```python
from build123d import *

# Parameters (mm, degrees)
SKETCH_1_R      = 1.5
SKETCH_1_R_2    = 5
EXTRUDE_1_DEPTH = 1


with BuildPart() as part:
    # 草图1 → 凸台-拉伸1 (new body)
    with BuildSketch(Plane.XY):
        with BuildLine():
            Line((-5, 25), (-5, -25))
            ThreePointArc((-5, -25), (0, -30), (5, -25))
            Line((5, -25), (5, 25))
            ThreePointArc((5, 25), (5.598988732, 30.259631636), (7.987721006, 34.983662814))
            ThreePointArc((7.987721006, 34.983662814), (0, 51), (-7.987721006, 34.983662814))
            ThreePointArc((-7.987721006, 34.983662814), (-5.598988732, 30.259631636), (-5, 25))
        make_face()
        with Locations((0, -25)):
            Circle(SKETCH_1_R, mode=Mode.SUBTRACT)
        with Locations((0, 25)):
            Circle(SKETCH_1_R, mode=Mode.SUBTRACT)
        with Locations((7.5, 41)):
            Circle(SKETCH_1_R, mode=Mode.SUBTRACT)
        with Locations((-7.5, 41)):
            Circle(SKETCH_1_R, mode=Mode.SUBTRACT)
        with Locations((0, 33.5)):
            Circle(SKETCH_1_R, mode=Mode.SUBTRACT)
        with Locations((0, 41)):
            Circle(SKETCH_1_R_2, mode=Mode.SUBTRACT)
        with Locations((0, 48.5)):
            Circle(SKETCH_1_R, mode=Mode.SUBTRACT)
    extrude(amount=EXTRUDE_1_DEPTH)


solid = part.part
```
The model under review builds one solid part; all positions refer to its coordinate system, in mm. Give positions to 0.01 mm unless a question says otherwise; leave off trailing zeros. Loops run counter-clockwise (first coordinate to the right, second up) from the corner with the lowest first, then second, coordinate; pieces in that order, holes last. Notation, with made-up numbers: (31.5, 22) -> (72.5, 22) arc R25 cw to (72.5, 39) -> close; hole circle Ø10 at (-27.75, 61). An arc over 180 degrees is marked (long way). Use CSV: the item, a comma, the result in double quotes.
1. Consider section D-D, the plane x = -3.75. Write out the cut boundary in (y, z).
Result:
outline,"(-28.31, 0) -> (37.69, 0) -> (37.69, 1) -> (-28.31, 1) -> close; (44.31, 0) -> (50.27, 0) -> (50.27, 1) -> (44.31, 1) -> close"
2. Consider section C-C, the plane z = 0.15. Write out the cut boundary in (x, y), then the cut area to 3 significant figures.
Result:
outline,"(-7.99, 34.98) arc R15 cw to (-5, 25) -> (-5, -25) arc R5 ccw to (5, -25) -> (5, 25) arc R15 cw to (7.99, 34.98) arc R10 ccw (long way) to start; hole circle Ø3 at (-7.5, 41); hole circle Ø10 at (0, 41); hole circle Ø3 at (0, -25); hole circle Ø3 at (0, 25); hole circle Ø3 at (0, 33.5); hole circle Ø3 at (0, 48.5); hole circle Ø3 at (7.5, 41)"
area,"805 mm²"
3. Consider section A-A, the plane x = 0. Write out the cut boundary in (y, z), then the cut area to 3 significant figures.
Result:
outline,"(-30, 0) -> (-26.5, 0) -> (-26.5, 1) -> (-30, 1) -> close; (-23.5, 0) -> (23.5, 0) -> (23.5, 1) -> (-23.5, 1) -> close; (26.5, 0) -> (32, 0) -> (32, 1) -> (26.5, 1) -> close; (35, 0) -> (36, 0) -> (36, 1) -> (35, 1) -> close; (46, 0) -> (47, 0) -> (47, 1) -> (46, 1) -> close; (50, 0) -> (51, 0) -> (51, 1) -> (50, 1) -> close"
area,"59.0 mm²"
4. To check wall thickness, follow probe 1 along X at (y, z) = (41.5, 0.4); probe 2 along X at (y, z) = (14.5, 0.8); probe 3 along Y at (x, z) = (-0.75, 0.15). State the ranges of each line that lie inside material, in increasing order. Write a range as from..to.
Result:
probe 1,"x = -9.99..-8.91, -6.09..-4.97, 4.97..6.09, 8.91..9.99"
probe 2,"x = -5..5"
probe 3,"y = -29.94..-26.3, -23.7..23.7, 26.3..32.2, 34.8..36.06, 45.94..47.2, 49.8..50.97"
5. Consider section B-B, the plane y = 48.5. Write out the cut boundary in (x, z).
Result:
outline,"(-6.61, 0) -> (-1.5, 0) -> (-1.5, 1) -> (-6.61, 1) -> close; (1.5, 0) -> (6.61, 0) -> (6.61, 1) -> (1.5, 1) -> close"
6. The part is to be moulded in two halves that separate along Y. For faces 1 (the face through (7.175, 39.536, 0.493)), 2 (the face through (0, 11, 1)), 3 (the face through (-7.825, 39.536, 0.493)), 4 (the face through (0.31, 50.995, 0.493)), say which applies: +Y half, -Y half, draft (parallel to the pull), parting line (faces both ways), or undercut.
Result:
face 1,"undercut"
face 2,"draft"
face 3,"undercut"
face 4,"parting line"
7. For P1, Ø0.5, axis at y = 12, z = 0.5, coming from the +X side, flat-tipped, find the tip position at first contact; note if it passes through.
Result:
P1,"stops at x = 5"
